Design review of the part built by this model. Coordinates are the model's own, in mm. Face numbers are marked on the shaded views. A direction names the side the tool comes from. Coordinates: 2 decimals unless noted, no trailing zeros. Loops run counter-clockwise (first coordinate to the right, second up) from the corner with the lowest first, then second, coordinate; pieces in that order, holes last. Notation, with made-up numbers: (43, 3.25) -> (49, 3.25) arc R24 ccw to (49, 34.25) -> close; hole circle Ø11 at (51.25, -13.5). An arc over 180 degrees is marked (long way). Use a Markdown table: item, result. Add a question column.
Q1. Draft analysis for pull direction X (two halves, no side actions). For the marked faces 1, 2 and 3, state which applies: pulls with the +X half, pulls with the -X half, needs draft (parallel to the pull), parting line crosses it, or undercut.
Q2. For probe 1 along X at (y, z) = (2.25, 15); probe 2 along Y at (x, z) = (0, 53.5) (3 decimals); probe 3 along Z at (x, y) = (1, 4.4), list the stretches that pass through material, from the lowest coordinate up.
Q3. Take a section at C-C on z = 6. Write out the cut boundary in (x, y).
Q4. For the marked faces 4, 5 and 6, list the 3-axis set-ups (+Z, -Z, +X, -X, +Y, -Y) from which the entire face can be reached by the end or side of a thin tool; tool diameter is ignored.
Q5. Clearance check with flat-ended pins moving along their axes: pin 1 Ø3 at (x, z) = (2.5, 26.5) entering from +Y; pin 2 Ø3 at (x, y) = (2.5, 4.5) entering from -Z. State where each tip first meets the part, or that it passes through.
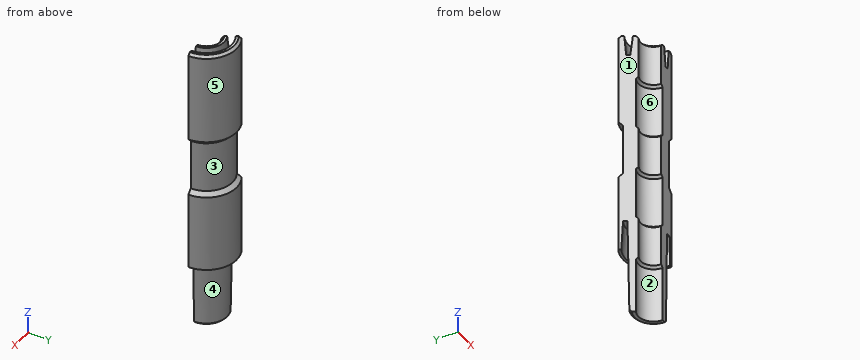
from build123d import *

# Parameters (mm, degrees)
REVOLVE_1_ANGLE = 120
CHAMFER_1_SIZE  = 0.4
CHAMFER_1_SIZE2 = 0.407145225
CHAMFER_2_SIZE  = 0.5


with BuildPart() as part:
    # 스케치1 → 회전1 (revolve)
    with BuildSketch(Plane(origin=(0, 0, 0), x_dir=(1, 0, 0), z_dir=(0, 1, 0))):
        Polygon((2.525, -30.375), (2.525, -38.375), (3, -38.85), (3, -48.85), (2.525, -49.325), (2.525, -57.325), (3, -57.8), (3.5, -57.8), (3.960399052, -53.8), (4.644221552, -53.8), (4.975, -57.8), (5.975, -57.8), (5.975, -39.8), (5.175, -39), (5.175, -29), (5.975, -28.2), (5.975, -13), (5.475, -13), (5.175, -19), (4.430616082, -19), (4.1, 0), (3, 0), (3, -10.95), (2.525, -11.425), (2.525, -19.425), (3, -19.9), (3, -29.9), align=None)
    revolve(axis=Axis((0, 0, 0), (0, 0, 1)), revolution_arc=REVOLVE_1_ANGLE)

    # 모따기1
    chamfer_1_edges = [part.edges().sort_by_distance(p)[0] for p in [
        (2.05, 3.550704156, 0),
    ]]
    chamfer_1_side = [part.faces().sort_by_distance(p)[0] for p in [
        (2.132654021, 3.693865118, 9.5),
    ]]
    chamfer(chamfer_1_edges, length=CHAMFER_1_SIZE, length2=CHAMFER_1_SIZE2, reference=chamfer_1_side[0])

    # 모따기2
    chamfer_2_edges = [part.edges().sort_by_distance(p)[0] for p in [
        (2.9875, 5.174501788, 57.8),
    ]]
    chamfer(chamfer_2_edges, length=CHAMFER_2_SIZE)


solid = part.part
Answer list:
| question | item | result |
|---|---|---|
| 1 | face 1 | pulls with the -X half |
| 1 | face 2 | undercut |
| 1 | face 3 | parting line crosses it |
| 2 | probe 1 | -1.3 to -1.15, 1.15 to 3.74, 4.88 to 5.54 |
| 2 | probe 2 | 2.525 to 5.975 |
| 2 | probe 3 | 19 to 53.8 |
| 3 | outline | (-2.1, 3.64) -> (-1.5, 2.6) arc R3 cw to (3, 0) -> (4.2, 0) arc R4.2 ccw to start |
| 4 | face 4 | -Z |
| 4 | face 5 | +Z, -Z, +Y |
| 4 | face 6 | -Y |
| 5 | pin 1 | y = 5.89 |
| 5 | pin 2 | z = 0 |
